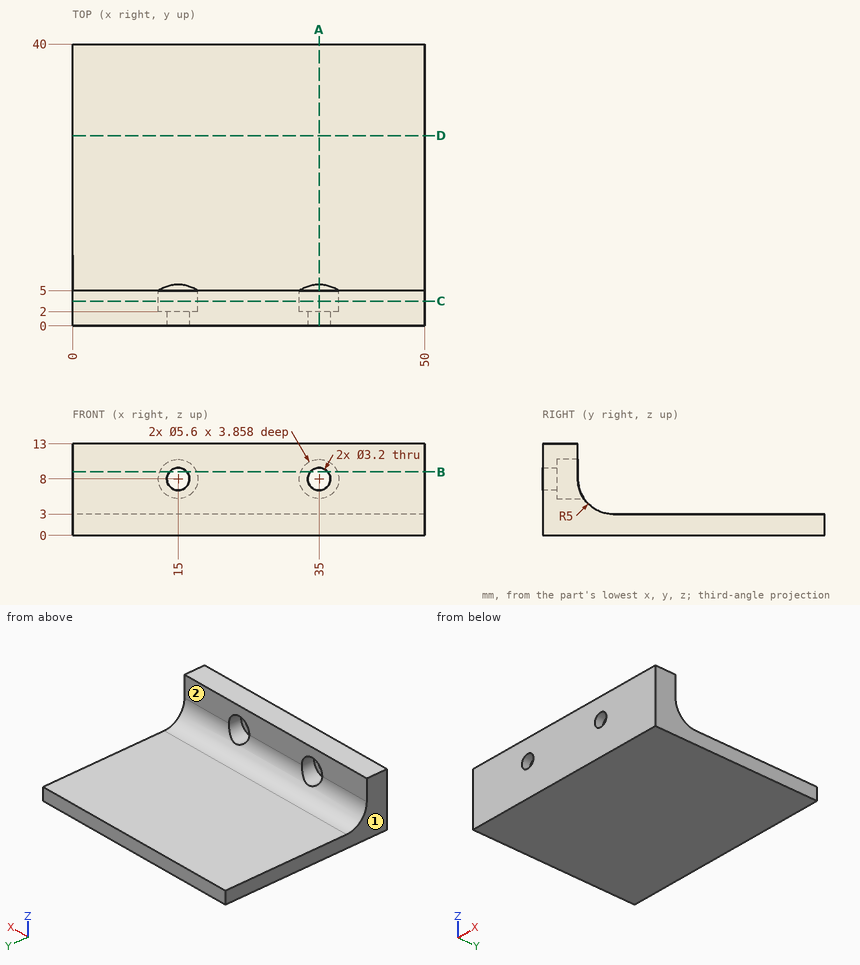
The drawing under review shows one solid part. Ordinate dimensions are in mm from its lowest x, y, z. A direction names the side the tool comes from. Coordinates: 2 decimals unless noted, no trailing zeros. Order: outer loops, then holes, each group sorted by start corner. A loop starts at its lowest first (then second) coordinate and runs counter-clockwise, first axis right, second up. Notation, with made-up numbers: (-35.75, 43) -> (-10.75, 43) arc R27 ccw to (-10.75, 61) -> close; hole circle Ø5 at (69, -24). An arc over 180 degrees is marked (long way). Return JSON: item names as keys, results as strings.
1. We need section A-A on x = 35. Write out the cut boundary in (y, z).
Answer block:
{"outline": "(0, 0) -> (40, 0) -> (40, 3) -> (10, 3) arc R5 cw to (5.86, 5.2) -> (2, 5.2) -> (2, 6.4) -> (0, 6.4) -> close; (0, 9.6) -> (2, 9.6) -> (2, 10.8) -> (5, 10.8) -> (5, 13) -> (0, 13) -> close"}
2. For pin 1 Ø6 at (x, y) = (44, 21) entering from +Z; pin 2 Ø6.5 at (x, z) = (35, 8) entering from -Y; pin 3 Ø5 at (x, z) = (39.5, 9.5) entering from +Y; pin 4 Ø1 at (x, z) = (12, 7) entering from +Y, all flat-tipped, find the tip position at first contact; note any pin that passes through.
Answer block:
{"pin 1": "z = 3", "pin 2": "y = 0", "pin 3": "y = 5.1", "pin 4": "y = 5.23"}
3. For line 1 (X direction, y = 1.1, z = 8); line 2 (Z direction, x = 21, y = 17); line 3 (Y direction, x = 6.5, z = 12.25), list the stretches that pass through material, from the lowest coordinate up. Write a range as from..to.
Answer block:
{"line 1": "0..13.4, 16.6..33.4, 36.6..50", "line 2": "0..3", "line 3": "0..5"}
4. Machinability: for the marked faces 1 and 2, which of the approach directions +Z, -Z, +X, -X, +Y, -Y give a long, thin tool a straight path to every point of the face, cutting with its end or side? Answer none if there is none.
Answer block:
{"face 1": "+Z, -Z, -X, +Y, -Y", "face 2": "+Z, +X, -X, +Y"}
5. We need section D-D on y = 27. Write out the cut boundary in (x, z), and give its area (3 significant figures).
Answer block:
{"outline": "(0, 0) -> (50, 0) -> (50, 3) -> (0, 3) -> close", "area": "150 mm²"}
6. We need section B-B on z = 9. Write out the cut boundary in (x, y) (1 decimal), and give its area (3 significant figures).
Answer block:
{"outline": "(0, 0) -> (13.8, 0) -> (13.8, 2) -> (12.4, 2) -> (12.4, 5) -> (0, 5) -> close; (16.2, 0) -> (33.8, 0) -> (33.8, 2) -> (32.4, 2) -> (32.4, 5) -> (17.6, 5) -> (17.6, 2) -> (16.2, 2) -> close; (36.2, 0) -> (50, 0) -> (50, 5) -> (37.6, 5) -> (37.6, 2) -> (36.2, 2) -> close", "area": "209 mm²"}
7. We need section C-C on y = 3.5. Write out the cut boundary in (x, z), and give its area (3 significant figures).
Answer block:
{"outline": "(0, 0) -> (50, 0) -> (50, 13) -> (0, 13) -> close; hole circle Ø5.6 at (15, 8); hole circle Ø5.6 at (35, 8)", "area": "601 mm²"}
